```python
from build123d import *

# Parameters (mm, degrees)
BOSS_EXTRU_1_DEPTH      = 20
ESQUISSE1_R             = 1
ENL_V_MAT_EXTRU_1_DEPTH = 4.4
BOSS_EXTRU_2_DEPTH      = 20
ESQUISSE3_R             = 1.25
ENL_V_MAT_EXTRU_2_DEPTH = 21


with BuildPart() as part:
    # ProfileRainureEsquisse → Boss.-Extru.1 (new body)
    with BuildSketch(Plane.XY):
        Polygon((0, 0), (0, 1.6), (1.8, 4.4), (1.8, 2.6), (3.4, 2.6), (3.4, -1), (1.8, -1), (1.8, -2.8), align=None)
    extrude(amount=BOSS_EXTRU_1_DEPTH)

    # Esquisse1 → Enlèv. mat.-Extru.1 (cut, through all)
    with BuildSketch(Plane(origin=(3.4, 0, 0), x_dir=(0, 0, -1), z_dir=(1, 0, 0))):
        with Locations((-5, 0.8)):
            Circle(ESQUISSE1_R)
    extrude(amount=-ENL_V_MAT_EXTRU_1_DEPTH, mode=Mode.SUBTRACT)

    # Esquisse2 → Boss.-Extru.2 (add)
    with BuildSketch(Plane(origin=(3.4, 0, 0), x_dir=(0, 0, -1), z_dir=(1, 0, 0))):
        Polygon((-16.6, 0), (-16.6, 1.6), (-18.4, 4.4), (-18.4, 2.6), (-20, 2.6), (-20, -1), (-18.4, -1), (-18.4, -2.8), align=None)
        Polygon((-11.4, 1.6), (-11.4, 0), (-9.6, -2.8), (-9.6, -1), (-8, -1), (-8, 2.6), (-9.6, 2.6), (-9.6, 4.4), align=None)
    extrude(amount=BOSS_EXTRU_2_DEPTH)

    # Esquisse3 → Enlèv. mat.-Extru.2 (cut, through all)
    with BuildSketch(Plane.XY.offset(20)):
        with Locations((18.4, 0.8)):
            Circle(ESQUISSE3_R)
    extrude(amount=-ENL_V_MAT_EXTRU_2_DEPTH, mode=Mode.SUBTRACT)


solid = part.part
```
Verification items for the finished model (mm, model axes). A direction names the side the tool comes from. Give positions to 0.01 mm unless a question says otherwise; leave off trailing zeros. Loops run counter-clockwise (first coordinate to the right, second up) from the corner with the lowest first, then second, coordinate; pieces in that order, holes last. Notation, with made-up numbers: M 53.25,88.5 L 65.25,88.5 A21 ccw 65.25,119.5 Z; hole C -34,46.5 d11. An arc over 180 degrees is marked long. Return JSON: item names as keys, results as strings.
1) Section check C-C, the plane z = 12.75. Enter the section's corners in (x, y), and give its area (3 significant figures).
Findings:
{"outline": "M 0,0 L 1.8,-2.8 L 1.8,-1 L 3.4,-1 L 3.4,2.6 L 1.8,2.6 L 1.8,4.4 L 0,1.6 Z", "area": "13.7 mm2"}
2) Mould release check, pull along X, two halves, no side actions. Record for faces 4 (the flat face through (0, 1, 13)), 5 (the flat face through (2, 1, 0)), 6 (the cylindrical face through (18.24, 2.04, 9.72)): released by +X, released by -X, zero draft, split by the parting line, or undercut.
Findings:
{"face 4": "released by -X", "face 5": "zero draft", "face 6": "undercut"}
3) Section check A-A, the plane x = 20.5. Enter the section's corners in (y, z).
Findings:
{"outline": "M -2.8,9.6 L -1,9.6 L -1,8 L 2.6,8 L 2.6,9.6 L 4.4,9.6 L 1.6,11.4 L 0,11.4 Z; M -2.8,18.4 L 0,16.6 L 1.6,16.6 L 4.4,18.4 L 2.6,18.4 L 2.6,20 L -1,20 L -1,18.4 Z"}
4) Tool access check on faces 1 (the flat face through (13.3, -1.4, 10.5)), 2 (the flat face through (13, -2, 18.4)), 3 (the flat face through (3.4, 1.2, 3.9)). Record the directions out of +Z, -Z, +X, -X, +Y, -Y that give a thin tool (end or side, any length) a straight path to the whole face; none if there is none.
Findings:
{"face 1": "+X, -Y", "face 2": "+Z, +X, -Y", "face 3": "-Z, +X, +Y, -Y"}
5) Material ranges on L1, parallel to X at y = 0.8, z = 8.7; L2, parallel to Z at x = 7.25, y = 0.5; L3, parallel to Y at x = 2.5, z = 10, recorded low to high. Write a range as [from, to].
Findings:
{"L1": "x = [0, 17.15], [19.65, 23.4]", "L2": "z = [8, 11.4], [16.6, 20]", "L3": "y = [-1, 2.6]"}
6) Section check B-B, the plane y = 0.8. Enter the section's corners in (x, z).
Findings:
{"outline": "M 0,0 L 3.4,0 L 3.4,4 L 0,4 Z; M 0,6 L 3.4,6 L 3.4,8 L 17.15,8 L 17.15,11.4 L 3.4,11.4 L 3.4,16.6 L 17.15,16.6 L 17.15,20 L 0,20 Z; M 19.65,8 L 23.4,8 L 23.4,11.4 L 19.65,11.4 Z; M 19.65,16.6 L 23.4,16.6 L 23.4,20 L 19.65,20 Z"}
7) Gauge pin test, flat ends, axial feed: P1, Ø1.3, axis at x = 21.5, y = 0.5, coming from the -Z side; P2, Ø0.9, axis at x = 15, y = -1.5, coming from the -Z side; P3, Ø3, axis at y = 0.5, z = 13, coming from the +X side. Record the tip position at first contact, or that the pin passes through.
Findings:
{"P1": "stops at z = 8", "P2": "stops at z = 9.6", "P3": "stops at x = 3.4"}
